from build123d import *

# Parameters (mm, degrees)
BOSS_EXTRUDE1_DEPTH = 26.9875
SKETCH2_R           = 2.0193
CUT_EXTRUDE1_DEPTH  = 19.05


with BuildPart() as part:
    # Sketch1 → Boss-Extrude1 (new, symmetric)
    with BuildSketch(Plane.XY):
        with BuildLine():
            ThreePointArc((4.7625, 1.891713919), (4.43790388, 2.562225), (4.019522311, 3.178589026))
            Line((4.019522311, 3.178589026), (0.742977689, 5.070302945))
            ThreePointArc((0.742977689, 5.070302945), (0, 5.12445), (-0.742977689, 5.070302945))
            Line((-0.742977689, 5.070302945), (-4.019522311, 3.178589026))
            ThreePointArc((-4.019522311, 3.178589026), (-4.43790388, 2.562225), (-4.7625, 1.891713919))
            Line((-4.7625, 1.891713919), (-4.7625, -1.891713919))
            ThreePointArc((-4.7625, -1.891713919), (-4.43790388, -2.562225), (-4.019522311, -3.178589026))
            Line((-4.019522311, -3.178589026), (-0.742977689, -5.070302945))
            ThreePointArc((-0.742977689, -5.070302945), (0, -5.12445), (0.742977689, -5.070302945))
            Line((0.742977689, -5.070302945), (4.019522311, -3.178589026))
            ThreePointArc((4.019522311, -3.178589026), (4.43790388, -2.562225), (4.7625, -1.891713919))
            Line((4.7625, -1.891713919), (4.7625, 1.891713919))
        make_face()
    extrude(amount=BOSS_EXTRUDE1_DEPTH, both=True)

    # Sketch2 → Cut-Extrude1 (cut)
    with BuildSketch(Plane(origin=(0, 0, -26.9875), x_dir=(-1, 0, 0), z_dir=(0, 0, -1))):
        Circle(SKETCH2_R)
    cut_extrude1 = extrude(amount=-CUT_EXTRUDE1_DEPTH, mode=Mode.SUBTRACT)

    # Mirror1: Cut-Extrude1 across plane
    add(cut_extrude1.mirror(Plane.XY), mode=Mode.SUBTRACT)


solid = part.part
Input: part model. Units: mm. Frame: model coordinates. A direction names the side the tool comes from. Coordinates: 2 decimals unless noted, no trailing zeros. Loops run counter-clockwise (first coordinate to the right, second up) from the corner with the lowest first, then second, coordinate; pieces in that order, holes last. Notation, with made-up numbers: (63.5, 36) -> (89.5, 36) arc R12 ccw to (89.5, 52) -> close; hole circle Ø8 at (-1.5, 77.25). An arc over 180 degrees is marked (long way). Write each question's results on one line, items separated by ' | '. Start each with the question number.
Q1. Pin query (flat end, axial travel): pin 1 (2 mm diameter, centred on x = -1, z = 18, fed in from +Y); pin 2 (3 mm diameter, centred on x = 0, y = 0, fed in from +Z); pin 3 (1 mm diameter, centred on x = -1.5, z = 14, fed in from -Y); pin 4 (1 mm diameter, centred on y = 3, z = -14.5, fed in from -X). Return the tip coordinate at first contact, or that it passes through.
Q2. Ray query, line 1 (Z direction, x = -1.75, y = 0.75); line 2 (Y direction, x = 4, z = -21.5); line 3 (Y direction, x = -1.75, z = -19.5). Return the intervals inside material, ascending. Write a range as from..to.
Q3. Reachability of faces 4 (the flat face through (0, 0, -7.938)), 5 (the cylindrical face through (-1.926, 0.607, 17.596)), 6 (the flat face through (-4.762, 0, 0)) from +Z, -Z, +X, -X, +Y, -Y: full face, straight path, thin tool, end or side. Return the list, or none.
Q4. Section C-C, the plane z = 6.5. Return the cut outline in (x, y), plus the area to 3 significant figures.
Q5. Pull-direction query (X, two-part tool) for faces 1 (the flat face through (-2.358, 4.138, 0.378)), 2 (the flat face through (2.404, 4.111, 0.378)), 3 (the cylindrical face through (-1.926, 0.607, -17.596)); classes: released by +X, released by -X, zero draft, split by the parting line, or undercut.
Q6. Section A-A, the plane z = 24.5. Return the cut outline in (x, y), plus the area to 3 significant figures.
Q7. Section B-B, the plane x = 0. Return the cut outline in (y, z), plus the area to 3 significant figures.
Q8. Section D-D, the plane y = -3.75. Return the cut outline in (x, z), plus the area to 3 significant figures.
Found:
1) pin 1: y = 5.12 | pin 2: z = 7.94 | pin 3: y = -4.92 | pin 4: x = -4.47
2) line 1: -7.94..7.94 | line 2: -3.19..3.19 | line 3: -4.49..-1.01, 1.01..4.49
3) face 4: -Z | face 5: +Z | face 6: +Z, -Z, -X, +Y, -Y
4) outline: (-4.76, -1.89) arc R5.12 ccw to (-4.02, -3.18) -> (-0.74, -5.07) arc R5.12 ccw to (0.74, -5.07) -> (4.02, -3.18) arc R5.12 ccw to (4.76, -1.89) -> (4.76, 1.89) arc R5.12 ccw to (4.02, 3.18) -> (0.74, 5.07) arc R5.12 ccw to (-0.74, 5.07) -> (-4.02, 3.18) arc R5.12 ccw to (-4.76, 1.89) -> close | area: 77.0 mm2
5) face 1: released by -X | face 2: released by +X | face 3: undercut
6) outline: (-4.76, -1.89) arc R5.12 ccw to (-4.02, -3.18) -> (-0.74, -5.07) arc R5.12 ccw to (0.74, -5.07) -> (4.02, -3.18) arc R5.12 ccw to (4.76, -1.89) -> (4.76, 1.89) arc R5.12 ccw to (4.02, 3.18) -> (0.74, 5.07) arc R5.12 ccw to (-0.74, 5.07) -> (-4.02, 3.18) arc R5.12 ccw to (-4.76, 1.89) -> close; hole circle Ø4.04 at (0, 0) | area: 64.2 mm2
7) outline: (-5.12, -26.99) -> (-2.02, -26.99) -> (-2.02, -7.94) -> (2.02, -7.94) -> (2.02, -26.99) -> (5.12, -26.99) -> (5.12, 26.99) -> (2.02, 26.99) -> (2.02, 7.94) -> (-2.02, 7.94) -> (-2.02, 26.99) -> (-5.12, 26.99) -> close | area: 399 mm2
8) outline: (-3.03, -26.99) -> (3.03, -26.99) -> (3.03, 26.99) -> (-3.03, 26.99) -> close | area: 327 mm2
